Autodesk Inventor part; units mm, degrees
ref_plane "housing_to_dummy_XY" through (0, 0, 0) normal (1, 0, 0) x (0, 0, -1)
ref_plane "housing_to_dummy_YZ" through (0, 0, 0) normal (0, 0, -1) x (0, 1, 0)
ref_plane "housing_to_dummy_ZX" through (0, 0, 0) normal (0, 1, 0) x (1, 0, 0)
sketch "Sketch_1" plane through (0, 0, 0) normal (0, 0, 1) x (1, 0, 0)
  line L0 (-36.5, -25) -> (-36.5, -40)
  line L1 (-36.5, -40) -> (36.5, -40)
  line L2 (36.5, -40) -> (36.5, -25)
  line L3 (36.5, -25) -> (22.5, -25)
  line L4 (22.5, -25) -> (22.5, 23)
  line L5 (22.5, 23) -> (-22.5, 23)
  line L6 (-22.5, 23) -> (-22.5, -25)
  line L7 (-22.5, -25) -> (-36.5, -25)
extrude "Extrusion1" add sketch "Sketch_1" along normal mid plane 15
sketch "Sketch2" plane through (0, 0, 7.5) normal (0, 0, 1) x (1, 0, 0)
  point P0 (0, 0)
hole "Hole1" at (0, 0, 7.5) direction (0, 0, -1) diameter 34 depth 15 counterbore diameter 37 counterbore depth 13
sketch "Sketch3" plane through (-36.5, -40, 7.5) normal (0, -1, 0) x (1, 0, 0)
  point P0 (7, -7.5)
hole "Hole2" at (-29.5, -40, 0) direction (0, 1, 0) diameter 6.5 depth 15
sketch "Sketch4" plane through (-36.5, -40, 7.5) normal (0, -1, 0) x (1, 0, 0)
  point P0 (66, -7.5)
hole "Hole3" at (29.5, -40, 0) direction (0, 1, 0) diameter 6.5 depth 15
sketch "Sketch_7" plane through (0, 0, 3.5) normal (0, 0, 1) x (1, 0, 0)
  circle A0 centre (0, 0) radius 19.9
extrude "Extrusion2" cut sketch "Sketch_7" along normal blind 1.6
sketch "Sketch6" plane through (0, 0, 7.5) normal (0, 0, 1) x (1, 0, 0)
  point P0 (-29.5, -32.5)
hole "Hole4" at (-29.5, -32.5, 7.5) direction (0, 0, -1) diameter 3.25 depth 0.02
ref_plane "housing_to_dummy_XY" through (0, 0, 0) normal (1, 0, 0) x (0, 0, -1)
ref_plane "housing_to_dummy_YZ" through (0, 0, 0) normal (0, 0, -1) x (0, 1, 0)
ref_plane "housing_to_dummy_ZX" through (0, 0, 0) normal (0, 1, 0) x (1, 0, 0)
ref_plane "to_bearing_XY" through (0, 0, -5.5) normal (0, 0, 1) x (1, 0, 0)
ref_plane "to_bearing_YZ" through (0, 0, -5.5) normal (1, 0, 0) x (0, 1, 0)
ref_plane "to_bearing_ZX" through (0, 0, -5.5) normal (0, 1, 0) x (0, 0, 1)
ref_plane "to_rring_XY" through (0, 0, 3.5) normal (0, 0, -1) x (1, 0, 0)
ref_plane "to_rring_YZ" through (0, 0, 3.5) normal (1, 0, 0) x (0, -1, 0)
ref_plane "to_rring_ZX" through (0, 0, 3.5) normal (0, -1, 0) x (0, 0, -1)
properties part number "BSHKSA6904ZZ-40_h"
Model file for the job. Use its own axes, mm. A direction names the side the tool comes from. Give positions to 0.01 mm unless a question says otherwise; leave off trailing zeros. Write each loop counter-clockwise with the first axis right and the second up, starting at its lowest first coordinate (ties: lowest second). Pieces come first, ordered by that corner, then holes. Notation, with made-up numbers: (-27, 73.25) - (14, 73.25) arc R23 cw to (14, 102.25) - close; hole circle Ø9 at (-2, -31). An arc over 180 degrees is marked (long way). One line per question, with ' | ' between items. Start each with the question number.
(1) 3-axis set-ups, long thin cutter, end or side, ignore diameter. For faces 4 (the face through (18.06, 4.01, 6.28)), 5 (the face through (-22.5, -1, 0)), 6 (the face through (6, -18, 5.1)), 7 (the face through (22.5, -1, 0)): which of +Z, -Z, +X, -X, +Y, -Y reach the whole face in a straight line?
(2) Slice it at A-A on z = 0. Write the cut outline in (x, y).
(3) Two-plate mould, pull along Z, no slides. Class faces 1 (the face through (-30, -32, 7.48)), 2 (the face through (-36.5, -32, 0)), 3 (the face through (6, -18, 3.5)): +Z half, -Z half, draft (parallel to the pull), parting line (faces both ways), or undercut.
(4) Slice it at D-D on z = 6. Write the cut outline in (x, y), plus the area to 3 significant figures.
(5) Slice it at C-C on y = 0. Write the cut outline in (x, z).
(6) Pin check, flat tips, straight feed: P1, Ø7.5, axis at y = 2, z = -2.5, coming from the -X side; P2, Ø2, axis at x = -24.5, z = -0.5, coming from the +Y side; P3, Ø1, axis at x = -29.5, y = -32, coming from the +Z side; P4, Ø4, axis at x = 28.5, z = 0, coming from the +Y side. Stop position of each tip, or through.
(7) Wall check: line 1 along X through (y, z) = (0, 6.55); line 2 along X through (y, z) = (0, -6.35); line 3 along Y through (x, z) = (0, 4.05). Give the ranges that are in metal, low to high. Write a range as from..to.
(8) Slice it at B-B on x = 29.5. Write the cut outline in (y, z), plus the area to 4 significant figures.
Results below:
1) face 4: +Z | face 5: +Z, -Z, -X, +Y | face 6: none | face 7: +Z, -Z, +X, +Y
2) outline: (-36.5, -40) - (-32.75, -40) - (-32.75, -25) - (-36.5, -25) - close; (-26.25, -40) - (26.25, -40) - (26.25, -25) - (22.5, -25) - (22.5, 23) - (-22.5, 23) - (-22.5, -25) - (-26.25, -25) - close; (32.75, -40) - (36.5, -40) - (36.5, -25) - (32.75, -25) - close; hole circle Ø37 at (0, 0)
3) face 1: +Z half | face 2: draft | face 3: undercut
4) outline: (-36.5, -40) - (36.5, -40) - (36.5, -25) - (22.5, -25) - (22.5, 23) - (-22.5, 23) - (-22.5, -25) - (-36.5, -25) - close; hole circle Ø37 at (0, 0) | area: 2,180 mm^2
5) outline: (-22.5, -7.5) - (-17, -7.5) - (-17, -5.5) - (-18.5, -5.5) - (-18.5, 3.5) - (-19.9, 3.5) - (-19.9, 5.1) - (-18.5, 5.1) - (-18.5, 7.5) - (-22.5, 7.5) - close; (17, -7.5) - (22.5, -7.5) - (22.5, 7.5) - (18.5, 7.5) - (18.5, 5.1) - (19.9, 5.1) - (19.9, 3.5) - (18.5, 3.5) - (18.5, -5.5) - (17, -5.5) - close
6) P1: x = -22.5 | P2: y = -25 | P3: z = 7.48 | P4: through
7) line 1: -22.5..-18.5, 18.5..22.5 | line 2: -22.5..-17, 17..22.5 | line 3: -40..-19.9, 19.9..23
8) outline: (-40, -7.5) - (-25, -7.5) - (-25, -3.25) - (-40, -3.25) - close; (-40, 3.25) - (-25, 3.25) - (-25, 7.5) - (-40, 7.5) - close | area: 127.5 mm^2
